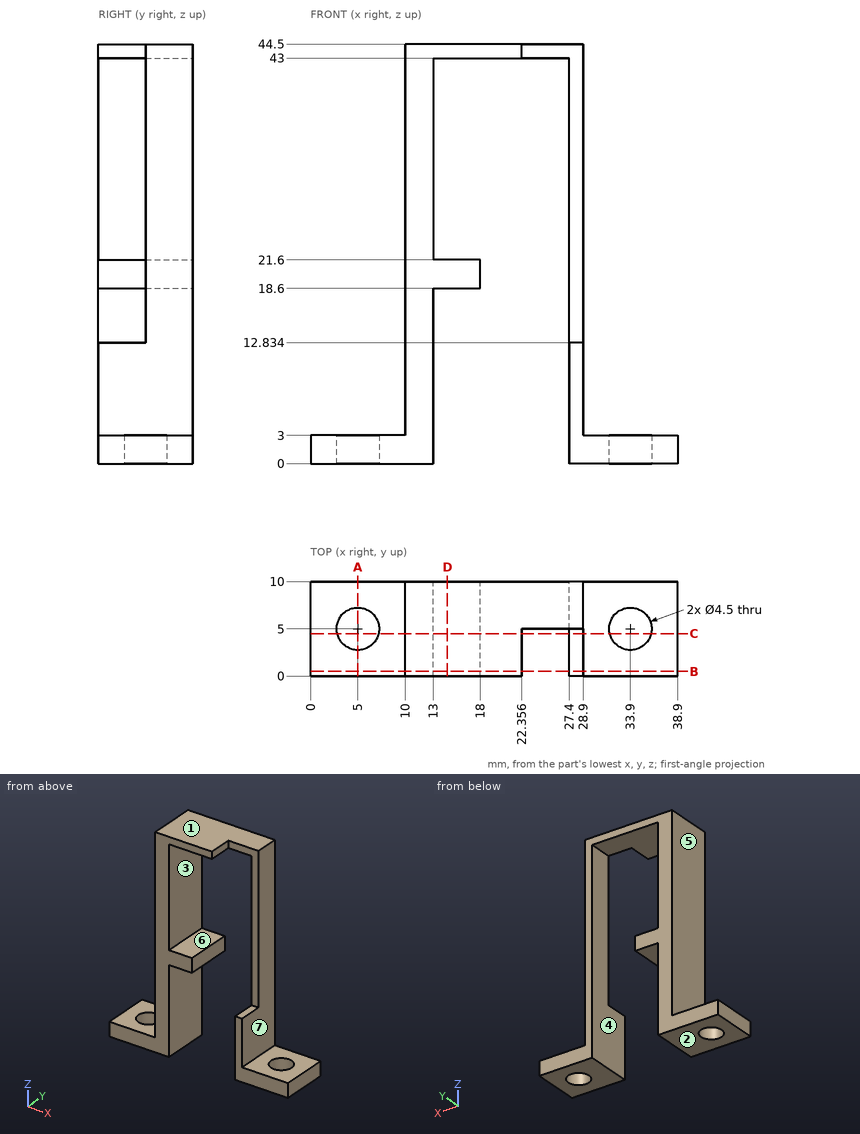
Job drawing, mm, ordinate dimensions from the low corner. One solid piece. A direction names the side the tool comes from. Coordinates: 2 decimals unless noted, no trailing zeros. Loops run counter-clockwise (first coordinate to the right, second up) from the corner with the lowest first, then second, coordinate; pieces in that order, holes last. Notation, with made-up numbers: (69, -8.75) -> (102, -8.75) arc R16 cw to (102, 17.25) -> close; hole circle Ø1 at (-12, 50). An arc over 180 degrees is marked (long way). One line per item, written item: value.
1. Flat gauge pins, fed straight in: P1, Ø2, axis at x = 27, z = 29, coming from the -Y side; P2, Ø4, axis at x = 6, y = 9, coming from the +Z side; P3, Ø1.6, axis at x = 28.5, y = 2.5, coming from the +Z side; P4, Ø2, axis at x = 8, z = 38, coming from the -Y side. Where does each tip first touch, or does it go through?
Answers:
P1: stops at y = 5
P2: stops at z = 3
P3: stops at z = 12.83
P4: passes through
2. Slice it at D-D on x = 14.5. Write the cut outline in (y, z).
Answers:
outline: (0, 18.6) -> (10, 18.6) -> (10, 21.6) -> (0, 21.6) -> close; (0, 43) -> (10, 43) -> (10, 44.5) -> (0, 44.5) -> close
3. Pull direction Z, two halves, no side cores. Call the marked faces 1, 2 and 3: pulls with the +Z half, pulls with the -Z half, needs draft (parallel to the pull), parting line crosses it, or undercut.
Answers:
face 1: pulls with the +Z half
face 2: pulls with the -Z half
face 3: undercut
4. Slice it at C-C on y = 4.5. Write the cut outline in (x, z) (1 decimal).
Answers:
outline: (0, 0) -> (2.8, 0) -> (2.8, 3) -> (0, 3) -> close; (7.2, 0) -> (13, 0) -> (13, 18.6) -> (18, 18.6) -> (18, 21.6) -> (13, 21.6) -> (13, 43) -> (22.4, 43) -> (22.4, 44.5) -> (10, 44.5) -> (10, 3) -> (7.2, 3) -> close; (27.4, 0) -> (31.7, 0) -> (31.7, 3) -> (28.9, 3) -> (28.9, 12.8) -> (27.4, 12.8) -> close; (36.1, 0) -> (38.9, 0) -> (38.9, 3) -> (36.1, 3) -> close
5. Slice it at B-B on y = 0.5. Write the cut outline in (x, z) (1 decimal).
Answers:
outline: (0, 0) -> (13, 0) -> (13, 18.6) -> (18, 18.6) -> (18, 21.6) -> (13, 21.6) -> (13, 43) -> (22.4, 43) -> (22.4, 44.5) -> (10, 44.5) -> (10, 3) -> (0, 3) -> close; (27.4, 0) -> (38.9, 0) -> (38.9, 3) -> (28.9, 3) -> (28.9, 12.8) -> (27.4, 12.8) -> close
6. Drill centre lines: line 1 (X direction, y = 7.25, z = 12.5); line 2 (Y direction, x = 33.9, z = 0.7); line 3 (Z direction, x = 9, y = 8). Where is each one in solid material? Low to high. Write a range as [from, to].
Answers:
line 1: x = [10, 13], [27.4, 28.9]
line 2: y = [0, 2.75], [7.25, 10]
line 3: z = [0, 3]
7. Slice it at A-A on x = 5. Write the cut outline in (y, z), and give its area (3 significant figures).
Answers:
outline: (0, 0) -> (2.75, 0) -> (2.75, 3) -> (0, 3) -> close; (7.25, 0) -> (10, 0) -> (10, 3) -> (7.25, 3) -> close
area: 16.5 mm^2
8. Which spindle directions (+Z, -Z, +X, -X, +Y, -Y) get a long thin tool onto all of the face, cutting with end or side? Do the marked faces 4, 5, 6 and 7. Say none if no direction does.
Answers:
face 4: -Z, +Y, -Y
face 5: +Z, -X, +Y, -Y
face 6: +Y, -Y
face 7: +Z, +X, +Y, -Y
